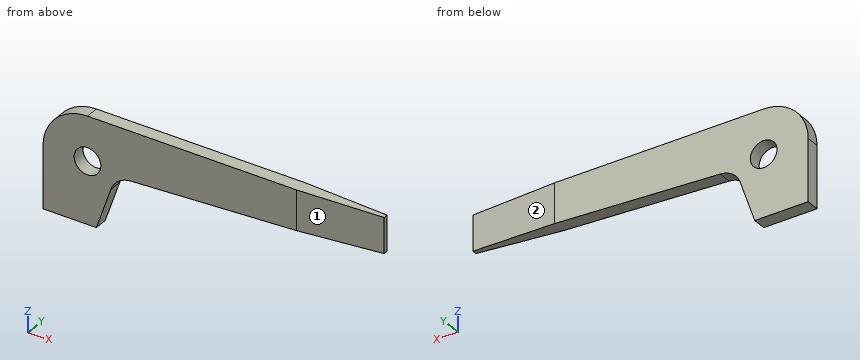
from build123d import *

# Parameters (mm, degrees)
F1_DEPTH = 2.38125
F2_R     = 2.38125
F3_DEPTH = 25.4
F5_DEPTH = 25.4


with BuildPart() as f1:
    # F0 (on Front) → F1 (new body)
    with BuildSketch(Plane.XZ):
        with BuildLine():
            Line((60.325, 19.05), (7.9375, 19.05))
            ThreePointArc((7.9375, 19.05), (2.32484, 16.72516), (0, 11.1125))
            Line((0, 11.1125), (0, 0))
            Line((0, 0), (9.525, 0))
            Line((9.525, 0), (12.117365, 7.627166))
            ThreePointArc((12.117365, 7.627166), (13.478615, 9.513592), (15.663196, 10.313094))
            Line((15.663196, 10.313094), (60.325, 12.7))
            Line((60.325, 12.7), (60.325, 19.05))
        make_face()
    extrude(amount=F1_DEPTH)

    # F2 (on face) → F3 (cut)
    with BuildSketch(Plane.XZ.offset(2.38125)):
        with Locations((7.9375, 11.1125)):
            Circle(F2_R)
    extrude(amount=-F3_DEPTH, mode=Mode.SUBTRACT)

    # F4 (on face) → F5 (cut)
    with BuildSketch(Plane.XY.offset(19.05)):
        Polygon((60.325, -2.38125), (60.325, -1.59385), (45.2374, -2.38125), align=None)
        Polygon((60.325, 0), (45.24375, 0), (60.325, -0.79375), align=None)
    extrude(amount=-F5_DEPTH, mode=Mode.SUBTRACT)


solid = f1.part
Could you check a few things on this model? Use its own coordinates, in mm. Face numbers are marked on the shaded views. Coordinates: 2 decimals unless noted, no trailing zeros. Order: outer loops, then holes, each group sorted by start corner. A loop starts at its lowest first (then second) coordinate and runs counter-clockwise, first axis right, second up.
Q1. Please list where these lines run through material, in increasing order: L1, parallel to Z at x = 45, y = -1; L2, parallel to X at y = -1.5, z = 13 (3 decimals); L3, parallel to Z at x = 6, y = -0.5.
Q2. Suppose I cut it at D-D on x = 16.5. Please give me the cut outline in (y, z).
Q3. Thinking about a two-plate mould opening in Y: for the marked faces 1 and 2, which applies, released by +Y, released by -Y, zero draft, split by the parting line, or undercut?
Q4. Suppose I cut it at C-C on z = 14.25. Please give me the cut outline in (x, y) (3 decimals).
Q5. Will these pins go through, and if not, where does the flat tip stop? pin 1 (5 mm diameter, centred on x = 53.5, z = 10, fed in from +Y); pin 2 (10 mm diameter, centred on x = 28, z = 2.5, fed in from -Y).
Q6. Suppose I cut it at B-B on x = 8.5. Please give me the cut outline in (y, z).
Answer:
1. L1: z = 11.88 to 19.05
1. L2: x = 0.228 to 6.486, 9.389 to 60.325
1. L3: z = 0 to 9.73, 12.5 to 18.81
2. outline: (-2.38, 10.36) - (0, 10.36) - (0, 19.05) - (-2.38, 19.05) - close
3. face 1: released by -Y
3. face 2: released by +Y
4. outline: (0.646, -2.381) - (45.237, -2.381) - (60.325, -1.594) - (60.325, -0.794) - (45.244, 0) - (0.646, 0) - close
5. pin 1: stops at y = -0.38
5. pin 2: passes through
6. outline: (-2.38, 0) - (0, 0) - (0, 8.8) - (-2.38, 8.8) - close; (-2.38, 13.43) - (0, 13.43) - (0, 19.05) - (-2.38, 19.05) - close
